Here's how the part is built. I have some questions about the finished solid (model axes, mm). Face numbers are marked on the shaded views. A direction names the side the tool comes from. Coordinates: 2 decimals unless noted, no trailing zeros. Write each loop counter-clockwise with the first axis right and the second up, starting at its lowest first coordinate (ties: lowest second). Pieces come first, ordered by that corner, then holes. Notation, with made-up numbers: (72, 37.25) -> (131, 37.25) arc R24 cw to (131, 58.25) -> close; hole circle Ø3 at (24.25, 64.25). An arc over 180 degrees is marked (long way). Put each result on its own line as item: value. Start each with the question number.
Item 1: I want a section at A-A, the plane x = -3.25. List the corners of the cut face in (y, z) for me.
Item 2: I need wall thicknesses on line 1 (X direction, y = 14.5, z = -2.75); line 2 (X direction, y = 2, z = -4.25); line 3 (Z direction, x = -4, y = 4.5). Which ranges of each line are inside material? Lowest first, please. Write a range as [from, to].
Item 3: If we mould it in two halves opening along X, with no side actions, what happens to the marked faces 3, 4, 5 and 6? For each: released by +X, released by -X, zero draft, split by the parting line, or undercut.
Item 4: I want a section at D-D, the plane x = -1.25. List the corners of the cut face in (y, z) for me, then the cut area to 3 significant figures.
Item 5: On a 3-axis mill with a long thin cutter (end or side, diameter ignored), from which of +Z, -Z, +X, -X, +Y, -Y can I reach the whole of each face in a straight line? I mean the marked faces 1 and 2. Say none if no direction works.
Item 6: I want a section at B-B, the plane y = 13.75. List the corners of the cut face in (x, z) for me, then the cut area to 3 significant figures.
Item 7: I want a section at C-C, the plane z = -4. List the corners of the cut face in (x, y) for me, then the cut area to 3 significant figures.
Item 8: For pin 1 (6 mm diameter, centred on y = 3.5, z = -9, fed in from -X); pin 2 (6 mm diameter, centred on x = -5.5, z = -9, fed in from -Y); pin 3 (1 mm diameter, centred on x = -4, y = 9.5, fed in from -Z); pin 4 (3 mm diameter, centred on y = 7.5, z = -8, fed in from -X), each with a flat end and sliding along its axis, tell me the tip position at first contact or that it passes through.
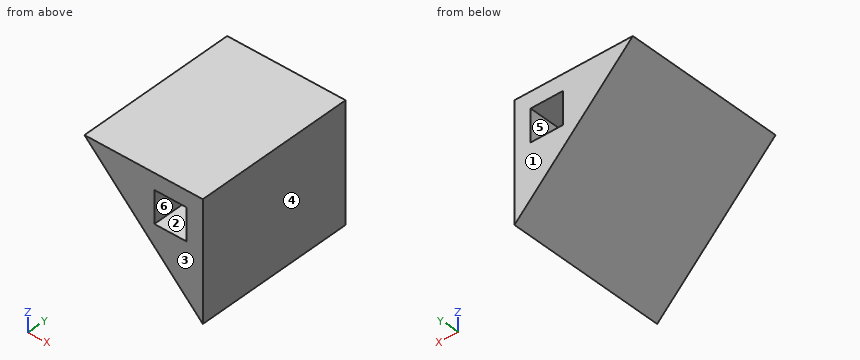
Autodesk Inventor part; units mm, degrees
ref_plane "YZ Plane" through (0, 0, 0) normal (1, 0, 0) x (0, 1, 0)
ref_plane "XZ Plane" through (0, 0, 0) normal (0, 1, 0) x (-1, 0, 0)
ref_plane "XY Plane" through (0, 0, 0) normal (0, 0, 1) x (1, 0, 0)
sketch "草圖1" plane through (0, 0, 0) normal (0, 1, 0) x (-1, 0, 0)
  line L0 (0, 0) -> (0, -11)
  line L1 (0, -11) -> (11, 0)
  line L2 (11, 0) -> (0, 0)
  line L3 (4.5, -1.5) -> (1.5, -1.5)
  line L4 (1.5, -1.5) -> (1.5, -4.5)
  line L5 (1.5, -4.5) -> (4.5, -4.5)
  line L6 (4.5, -4.5) -> (4.5, -1.5)
  dimension "d0" = 11
  dimension "d1" = 11
  dimension "d4" = 3
  dimension "d5" = 3
  dimension "d8" = 1.5
  dimension "d9" = 1.5
extrude "擠出1" add sketch "草圖1" along normal blind 15
properties part number "triangle"
Calculated:
1. outline: (0, -7.75) -> (15, -7.75) -> (15, -4.5) -> (0, -4.5) -> close; (0, -1.5) -> (15, -1.5) -> (15, 0) -> (0, 0) -> close
2. line 1: x = [-8.25, -4.5], [-1.5, 0]
2. line 2: x = [-6.75, -4.5], [-1.5, 0]
2. line 3: z = [-7, -4.5], [-1.5, 0]
3. face 3: zero draft
3. face 4: released by +X
3. face 5: undercut
3. face 6: undercut
4. outline: (0, -9.75) -> (15, -9.75) -> (15, 0) -> (0, 0) -> close
4. area: 146 mm2
5. face 1: +Z, -Z, +X, -X, +Y
5. face 2: +Y, -Y
6. outline: (-11, 0) -> (0, -11) -> (0, 0) -> close; hole (-4.5, -4.5) -> (-1.5, -4.5) -> (-1.5, -1.5) -> (-4.5, -1.5) -> close
6. area: 51.5 mm2
7. outline: (-7, 0) -> (-4.5, 0) -> (-4.5, 15) -> (-7, 15) -> close; (-1.5, 0) -> (0, 0) -> (0, 15) -> (-1.5, 15) -> close
7. area: 60.0 mm2
8. pin 1: stops at x = -5
8. pin 2: stops at y = 0
8. pin 3: stops at z = -7.5
8. pin 4: stops at x = -4.5
